Check sheet for the modelled part. Datum: model origin and axes. Units: mm. Coordinates: 2 decimals unless noted, no trailing zeros. Loops run counter-clockwise (first coordinate to the right, second up) from the corner with the lowest first, then second, coordinate; pieces in that order, holes last. Notation, with made-up numbers: (7.25, 58) - (29.25, 58) arc R23 cw to (29.25, 82) - close; hole circle Ø7 at (-0.5, 10.25). An arc over 180 degrees is marked (long way). Write each question's results on one line, items separated by ' | '. Start each with the question number.
1. Cross-section at A-A (z = 655.5). Record the cut outline in (x, y).
2. Thickness scan on line 1 (Y direction, x = -4.4, z = 776); line 2 (Z direction, x = -4, y = 4.25); line 3 (X direction, y = 4.5, z = 414). Record the ranges inside material, lowest first. Write a range as [from, to].
3. Draft check along X on faces 1 (the face through (-5, 0, 385)), 2 (the face through (3.5, 0, 385)), 3 (the face through (5, 0, 385)). Enter one of: released by +X, released by -X, zero draft, split by the parting line, or undercut.
```python
from build123d import *

# Parameters (mm, degrees)
SKETCH_1_W          = 10
SKETCH_1_H          = 15
SKETCH_1_W_2        = 7
SKETCH_1_H_2        = 12
EXTRUDE_1_DEPTH     = 781
SKETCH_2_R          = 2
SKETCH_2_R_2        = 1.5
CUT_EXTRUDE_1_DEPTH = 782.100025605
SKETCH_3_R          = 2
SKETCH_3_R_2        = 1.5
CUT_EXTRUDE_2_DEPTH = 782.16003482


with BuildPart() as part:
    # ｽｹｯﾁ1 → 押し出し-薄板1 (new body)
    with BuildSketch(Plane.XY):
        Rectangle(SKETCH_1_W, SKETCH_1_H)
        Rectangle(SKETCH_1_W_2, SKETCH_1_H_2, mode=Mode.SUBTRACT)
    extrude(amount=EXTRUDE_1_DEPTH)

    # ｽｹｯﾁ2 → ｶｯﾄ - 押し出し1 (cut, through all)
    with BuildSketch(Plane(origin=(5, 0, 0), x_dir=(0, 0, -1), z_dir=(1, 0, 0))):
        with Locations((-470, 0)):
            Circle(SKETCH_2_R)
        with Locations((-450, 0)):
            Circle(SKETCH_2_R)
        with Locations((-15, 4)):
            Circle(SKETCH_2_R_2)
        with Locations((-15, -4)):
            Circle(SKETCH_2_R_2)
        with Locations((-776, 4)):
            Circle(SKETCH_2_R_2)
        with Locations((-776, -4)):
            Circle(SKETCH_2_R_2)
    extrude(amount=-CUT_EXTRUDE_1_DEPTH, mode=Mode.SUBTRACT)

    # ｽｹｯﾁ3 → ｶｯﾄ - 押し出し2 (cut, through all)
    with BuildSketch(Plane(origin=(0, 7.5, 0), x_dir=(1, 0, 0), z_dir=(0, 1, 0))):
        with Locations(Location((0, -5, 0), (0, 0, 270))):
            Circle(SKETCH_3_R)
        with Locations(Location((0, -764.5, 0), (0, 0, 270))):
            Circle(SKETCH_3_R_2)
    extrude(amount=-CUT_EXTRUDE_2_DEPTH, mode=Mode.SUBTRACT)


solid = part.part
```
Established:
1) outline: (-5, -7.5) - (5, -7.5) - (5, 7.5) - (-5, 7.5) - close; hole (-3.5, -6) - (3.5, -6) - (3.5, 6) - (-3.5, 6) - close
2) line 1: [-7.5, -5.5], [-2.5, 2.5], [5.5, 7.5] | line 2: [0, 13.52], [16.48, 774.52], [777.48, 781] | line 3: [-5, -3.5], [3.5, 5]
3) face 1: released by -X | face 2: undercut | face 3: released by +X
